For this review, take the finished solid that the model builds, in its own axes (mm). A direction names the side the tool comes from. Give positions to 0.01 mm unless a question says otherwise; leave off trailing zeros. Loops run counter-clockwise (first coordinate to the right, second up) from the corner with the lowest first, then second, coordinate; pieces in that order, holes last.
```python
from build123d import *

# Parameters (mm, degrees)
SKETCH1_R           = 76.2
SKETCH1_R_2         = 4.7625
BOSS_EXTRUDE1_DEPTH = 6.35
SKETCH2_R           = 12.7
BOSS_EXTRUDE2_DEPTH = 76.2
SKETCH3_R           = 12.7
SKETCH3_R_2         = 9.525
CUT_EXTRUDE1_DEPTH  = 12.7
SKETCH4_R           = 3
CUT_EXTRUDE2_DEPTH  = 86.725


with BuildPart() as part:
    # Sketch1 → Boss-Extrude1 (new body)
    with BuildSketch(Plane.XY):
        Circle(SKETCH1_R)
        with Locations((0, 50.8)):
            Circle(SKETCH1_R_2, mode=Mode.SUBTRACT)
        with Locations((43.994090512, 25.4)):
            Circle(SKETCH1_R_2, mode=Mode.SUBTRACT)
        with Locations((43.994090512, -25.4)):
            Circle(SKETCH1_R_2, mode=Mode.SUBTRACT)
        with Locations((0, -50.8)):
            Circle(SKETCH1_R_2, mode=Mode.SUBTRACT)
        with Locations((-43.994090512, -25.4)):
            Circle(SKETCH1_R_2, mode=Mode.SUBTRACT)
        with Locations((-43.994090512, 25.4)):
            Circle(SKETCH1_R_2, mode=Mode.SUBTRACT)
    extrude(amount=BOSS_EXTRUDE1_DEPTH)

    # Sketch2 → Boss-Extrude2 (add)
    with BuildSketch(Plane.XY.offset(6.35)):
        Circle(SKETCH2_R)
    extrude(amount=BOSS_EXTRUDE2_DEPTH)

    # Sketch3 → Cut-Extrude1 (cut)
    with BuildSketch(Plane.XY.offset(82.55)):
        Circle(SKETCH3_R)
        Circle(SKETCH3_R_2, mode=Mode.SUBTRACT)
    extrude(amount=-CUT_EXTRUDE1_DEPTH, mode=Mode.SUBTRACT)

    # Sketch4 → Cut-Extrude2 (cut, through all)
    with BuildSketch(Plane(origin=(9.525, 0, 0), x_dir=(0, 0, -1), z_dir=(1, 0, 0))):
        with Locations((-76.2, 0)):
            Circle(SKETCH4_R)
    extrude(amount=-CUT_EXTRUDE2_DEPTH, mode=Mode.SUBTRACT)


solid = part.part
```
Q1. For pin 1 Ø10 at (x, y) = (-17, 43) entering from +Z; pin 2 Ø8 at (y, z) = (1.5, 42) entering from -X; pin 3 Ø6 at (x, z) = (47.5, 9) entering from +Y, all flat-tipped, find the tip position at first contact; note any pin that passes through.
Answers:
pin 1: stops at z = 6.35
pin 2: stops at x = -12.7
pin 3: stops at y = 60.68
Q2. Consider section A-A on x = 0. Count the separate pieces of the cut face and the enclosed holes in it, plus the area to 3 significant figures.
Answers:
separate pieces: 3
enclosed holes: 1
area: 2,670 mm2
Q3. Consider section B-B on y = 0. Give the boundary of the cut face in (x, z) (3 decimals).
Answers:
outline: (-76.2, 0) - (76.2, 0) - (76.2, 6.35) - (12.7, 6.35) - (12.7, 69.85) - (9.525, 69.85) - (9.525, 73.2) - (-9.525, 73.2) - (-9.525, 69.85) - (-12.7, 69.85) - (-12.7, 6.35) - (-76.2, 6.35) - close; (-9.525, 79.2) - (9.525, 79.2) - (9.525, 82.55) - (-9.525, 82.55) - close
Q4. Mouldability with a two-part tool opening along Z and no side actions: class faces 3 (the cylindrical face through (0.13, 0.9, 73.34)), 4 (the flat face through (5, 9, 69.85)), 5 (the cylindrical face through (-3.51, 54.02, 3.13)), 6 (the flat face through (-1, 1, 0)) as +Z half, -Z half, draft (parallel to the pull), parting line (faces both ways), or undercut.
Answers:
face 3: undercut
face 4: +Z half
face 5: draft
face 6: -Z half
Q5. Consider section C-C on y = -25.4. Give the boundary of the cut face in (x, z), plus the area to 3 significant figures.
Answers:
outline: (-71.84, 0) - (-48.76, 0) - (-48.76, 6.35) - (-71.84, 6.35) - close; (-39.23, 0) - (39.23, 0) - (39.23, 6.35) - (-39.23, 6.35) - close; (48.76, 0) - (71.84, 0) - (71.84, 6.35) - (48.76, 6.35) - close
area: 791 mm2
Q6. Machinability: for faces 1 (the cylindrical face through (8.8, -3.65, 76.29)), 2 (the cylindrical face through (48.537, 26.831, 3.131)), which of the approach directions +Z, -Z, +X, -X, +Y, -Y give a long, thin tool a straight path to every point of the face, cutting with its end or side? Answer none if there is none.
Answers:
face 1: +Z
face 2: +Z, -Z
Q7. Consider section D-D on z = 76.2. Give the boundary of the cut face in (x, y) (3 decimals).
Answers:
outline: (-9.04, -3) arc R9.525 ccw to (9.04, -3) - close; (-9.04, 3) - (9.04, 3) arc R9.525 ccw to start
Q8. For probe 1 along X at (y, z) = (-25, 4); probe 2 along Z at (x, y) = (24.5, 59.5); probe 3 along X at (y, z) = (50, 3), list the stretches that pass through material, from the lowest coordinate up.
Answers:
probe 1: x = -71.98 to -48.74, -39.25 to 39.25, 48.74 to 71.98
probe 2: z = 0 to 6.35
probe 3: x = -57.5 to -4.69, 4.69 to 57.5
